```python
from build123d import *

# Parameters (mm, degrees)
SKETCH1_W           = 20
SKETCH1_H           = 9
BOSS_EXTRUDE1_DEPTH = 13
CUT_EXTRUDE1_DEPTH  = 3
FILLET1_R           = 3


with BuildPart() as part:
    # Sketch1 → Boss-Extrude1 (new body)
    with BuildSketch(Plane.XY):
        Rectangle(SKETCH1_W, SKETCH1_H)
    extrude(amount=BOSS_EXTRUDE1_DEPTH)

    # Sketch2 → Cut-Extrude1 (cut)
    with BuildSketch(Plane.XY.offset(13)):
        with BuildLine():
            Line((1.51, -4.5), (1.51, -4.099981132))
            ThreePointArc((1.51, -4.099981132), (0, 1.6), (-1.51, -4.099981132))
            Line((-1.51, -4.099981132), (-1.51, -4.5))
            Line((-1.51, -4.5), (1.51, -4.5))
        make_face()
    extrude(amount=-CUT_EXTRUDE1_DEPTH, mode=Mode.SUBTRACT)

    # Fillet1
    fillet1_edges = [part.edges().sort_by_distance(p)[0] for p in [
        (-10, 4.5, 6.5),
        (10, 4.5, 6.5),
    ]]
    fillet(fillet1_edges, radius=FILLET1_R)


solid = part.part
```
Geometry check sheet. Reference: the model listing, model coordinates, mm. Give positions to 0.01 mm unless a question says otherwise; leave off trailing zeros. Order: outer loops, then holes, each group sorted by start corner. A loop starts at its lowest first (then second) coordinate and runs counter-clockwise, first axis right, second up. Notation, with made-up numbers: (-29, 36) - (22, 36) arc R10 cw to (22, 48) - close; hole circle Ø10 at (63, -29.75). An arc over 180 degrees is marked (long way). Write item = value, one per line. Start each with the question number.
1) Section check C-C (x = 2.75). Enter the section's corners in (y, z), then the cut area to 3 significant figures.
2) Draft check along X on faces 1 (the flat face through (0, 4.5, 6)), 2 (the cylindrical face through (0.1, 1.6, 11.5)), 3 (the flat face through (0, -1, 10)), 4 (the flat face through (-10, -2, 6)). Enter one of: released by +X, released by -X, zero draft, split by the parting line, or undercut.
3) Section check A-A (y = -1.45). Enter the section's corners in (x, z).
4) Section check D-D (z = 5.25). Enter the section's corners in (x, y).
5) Scan lines: L1, parallel to X at y = -1.45, z = 11.35; L2, parallel to Z at x = -0.25, y = -1.25; L3, parallel to Y at x = 0, z = 11.4. Record each from-to range of solid material in increasing order.
6) Section check B-B (z = 11). Enter the section's corners in (x, y), then the cut area to 3 significant figures.
Geometry check:
q1.outline = (-4.5, 0) - (4.5, 0) - (4.5, 13) - (-0.13, 13) - (-0.13, 10) - (-2.77, 10) - (-2.77, 13) - (-4.5, 13) - close
q1.area = 109 mm2
q2.face_1 = zero draft
q2.face_2 = undercut
q2.face_3 = undercut
q2.face_4 = released by -X
q3.outline = (-10, 0) - (10, 0) - (10, 13) - (3.05, 13) - (3.05, 10) - (-3.05, 10) - (-3.05, 13) - (-10, 13) - close
q4.outline = (-10, -4.5) - (10, -4.5) - (10, 1.5) arc R3 ccw to (7, 4.5) - (-7, 4.5) arc R3 ccw to (-10, 1.5) - close
q5.L1 = -10 to -3.05, 3.05 to 10
q5.L2 = 0 to 10
q5.L3 = 1.6 to 4.5
q6.outline = (-10, -4.5) - (-1.51, -4.5) - (-1.51, -4.1) arc R3.05 cw (long way) to (1.51, -4.1) - (1.51, -4.5) - (10, -4.5) - (10, 1.5) arc R3 ccw to (7, 4.5) - (-7, 4.5) arc R3 ccw to (-10, 1.5) - close
q6.area = 147 mm2
